```python
from build123d import *

# Parameters (mm, degrees)
F0_W     = 230
F0_H     = 200
F1_DEPTH = 25
F2_W     = 5
F2_H     = 20
F2_R     = 1.5
F3_DEPTH = 25
F4_DEPTH = 25


with BuildPart() as f1:
    # F0 (on Front) → F1 (new body)
    with BuildSketch(Plane.XZ):
        with Locations((-169.041439, -113.966247)):
            Rectangle(F0_W, F0_H)
    extrude(amount=F1_DEPTH)

    # F2 (on face) → F3 (cut)
    with BuildSketch(Plane.XZ.offset(25)):
        with Locations((-271.541439, -73.966247)):
            Rectangle(F2_W, F2_H)
        with Locations((-79.041439, -40.466247)):
            Circle(F2_R)
        with Locations((-79.041439, -187.466247)):
            Circle(F2_R)
        with Locations((-259.041439, -38.966247)):
            Circle(F2_R)
        with Locations((-259.041439, -188.966247)):
            Circle(F2_R)
    extrude(amount=-F3_DEPTH, mode=Mode.SUBTRACT)

    # F2 (on face) → F4 (cut)
    with BuildSketch(Plane.XZ.offset(25)):
        with Locations((-271.541439, -73.966247)):
            Rectangle(F2_W, F2_H)
        with Locations((-79.041439, -40.466247)):
            Circle(F2_R)
        with Locations((-79.041439, -187.466247)):
            Circle(F2_R)
        with Locations((-259.041439, -38.966247)):
            Circle(F2_R)
        with Locations((-259.041439, -188.966247)):
            Circle(F2_R)
    extrude(amount=-F4_DEPTH, mode=Mode.SUBTRACT)


solid = f1.part
```
Source: CAD feature listing. Evaluate the final solid. Frame: model axes, mm. A direction names the side the tool comes from. Give positions to 0.01 mm unless a question says otherwise; leave off trailing zeros. Use a Markdown table: item, result. Add a question column.
(1) Access query for faces 1 (the face through (-272, -13, -63.966)), 2 (the face through (-171, -25, -113)). Directions: +Z, -Z, +X, -X, +Y, -Y. A direction counts if a zero-diameter tool reaches every point of the face in a straight line with its end or side. Return the directions, or none.
(2) First-contact query: pin 1 Ø2.5 at (x, z) = (-79.04, -187.47) entering from +Y. Flat tip, straight axial feed; report the tip coordinate or a pass-through.
(3) Ray query, line 1 (X direction, y = -19.25, z = -78); line 2 (Z direction, x = -260, y = -8). Return the intervals inside material, ascending.
(4) Pull-direction query (Z, two-part tool) for faces 3 (the face through (-171, 0, -113)), 4 (the face through (-171, -12, -213.966)), 5 (the face through (-274.041, -13, -74)), 6 (the face through (-171, -12, -13.966)); classes: +Z half, -Z half, draft (parallel to the pull), parting line (faces both ways), or undercut.
Checked values:
| question | item | result |
|---|---|---|
| 1 | face 1 | +Y, -Y |
| 1 | face 2 | +Z, -Z, +X, -X, -Y |
| 2 | pin 1 | through |
| 3 | line 1 | -284.04 to -274.04, -269.04 to -54.04 |
| 3 | line 2 | -213.97 to -190.12, -187.81 to -40.12, -37.81 to -13.97 |
| 4 | face 3 | draft |
| 4 | face 4 | -Z half |
| 4 | face 5 | undercut |
| 4 | face 6 | +Z half |
